Source: CAD feature listing. Evaluate the final solid. Frame: model axes, mm. Coordinates: 2 decimals unless noted, no trailing zeros. Loops run counter-clockwise (first coordinate to the right, second up) from the corner with the lowest first, then second, coordinate; pieces in that order, holes last. Notation, with made-up numbers: (-13, -18) - (20, -18) arc R15 ccw to (20, 7) - close; hole circle Ø9 at (-32, 53). An arc over 180 degrees is marked (long way). Use one line per item in the form item = value. Start each with the question number.
from build123d import *

# Parameters (mm, degrees)
SKETCH1_W           = 7.75
SKETCH1_H           = 9.75
BOSS_EXTRUDE1_DEPTH = 50
SKETCH4_R           = 2
CUT_EXTRUDE3_DEPTH  = 9.75
CHAMFER1_SIZE       = 0.5


with BuildPart() as part:
    # Sketch1 → Boss-Extrude1 (new body)
    with BuildSketch(Plane(origin=(0, 0, 0), x_dir=(0, 0, -1), z_dir=(1, 0, 0))):
        with Locations((3.875, 4.875)):
            Rectangle(SKETCH1_W, SKETCH1_H)
    extrude(amount=BOSS_EXTRUDE1_DEPTH)

    # Sketch4 → Cut-Extrude3 (cut)
    with BuildSketch(Plane(origin=(0, 9.75, 0), x_dir=(1, 0, 0), z_dir=(0, 1, 0))):
        with Locations((3, 3.875)):
            Circle(SKETCH4_R)
        with Locations((45.75, 3.875)):
            Circle(SKETCH4_R)
    extrude(amount=-CUT_EXTRUDE3_DEPTH, mode=Mode.SUBTRACT)

    # Chamfer1
    chamfer1_edges = [part.edges().sort_by_distance(p)[0] for p in [
        (50, 4.875, -7.75),
        (50, 9.75, -3.875),
        (50, 4.875, 0),
        (0, 9.75, -3.875),
        (0, 4.875, -7.75),
        (0, 0, -3.875),
        (0, 4.875, 0),
        (25, 9.75, 0),
        (25, 9.75, -7.75),
        (25, 0, -7.75),
        (25, 0, 0),
        (50, 0, -3.875),
    ]]
    chamfer(chamfer1_edges, length=CHAMFER1_SIZE)


solid = part.part
(1) Material intervals for line 1 (Z direction, x = 3, y = 4.25) (3 decimals); line 2 (X direction, y = 6.5, z = -3.5); line 3 (X direction, y = 7, z = -4.75), sorted ascending.
(2) Cut plane B-B, the plane y = 6.75. Output: boundary loops of the cut face in (x, z) (3 decimals).
(3) Mould query, pull axis X, two halves, no side actions, for faces 1 (the face through (2.57, 4.94, -1.92)), 2 (the face through (0, 5, -4)), 3 (the face through (25, 0, -4)). Classes: +X half, -X half, draft (parallel to the pull), parting line (faces both ways), or undercut.
(4) Cut plane C-C, the plane z = -5. Output: boundary loops of the cut face in (x, y), plus the area to 3 significant figures.
(5) Cut plane A-A, the plane x = 3. Output: boundary loops of the cut face in (y, z) (3 decimals), plus the area to 3 significant figures.
Recorded:
q1.line_1 = -7.75 to -5.875, -1.875 to 0
q1.line_2 = 0 to 1.04, 4.96 to 43.79, 47.71 to 50
q1.line_3 = 0 to 1.2, 4.8 to 43.95, 47.55 to 50
q2.outline = (0, -7.25) - (0.5, -7.75) - (49.5, -7.75) - (50, -7.25) - (50, -0.5) - (49.5, 0) - (0.5, 0) - (0, -0.5) - close; hole circle Ø4 at (3, -3.875); hole circle Ø4 at (45.75, -3.875)
q3.face_1 = undercut
q3.face_2 = -X half
q3.face_3 = draft
q4.outline = (0, 0.5) - (0.5, 0) - (1.35, 0) - (1.35, 9.75) - (0.5, 9.75) - (0, 9.25) - close; (4.65, 0) - (44.1, 0) - (44.1, 9.75) - (4.65, 9.75) - close; (47.4, 0) - (49.5, 0) - (50, 0.5) - (50, 9.25) - (49.5, 9.75) - (47.4, 9.75) - close
q4.area = 423 mm²
q5.outline = (0, -7.25) - (0.5, -7.75) - (9.25, -7.75) - (9.75, -7.25) - (9.75, -5.875) - (0, -5.875) - close; (0, -1.875) - (9.75, -1.875) - (9.75, -0.5) - (9.25, 0) - (0.5, 0) - (0, -0.5) - close
q5.area = 36.1 mm²
